from build123d import *

# Parameters (mm, degrees)
SKETCH1_R           = 7.5
BOSS_EXTRUDE1_DEPTH = 60
CUT_EXTRUDE2_DEPTH  = 60
SKETCH3_R           = 7
CUT_EXTRUDE3_DEPTH  = 104.406963015
CHAMFER1_SIZE       = 15
SPLIT2_START        = 46
SPLIT2_OUTLINE_R    = 7.5
SPLIT2_DEPTH        = 14
SPLIT2_START_2      = 52
SPLIT2_2_DEPTH      = 8
SPLIT2_3_DEPTH      = 58
SHELL1_START        = 48
SHELL1_DEPTH        = 12
SHELL1_START_2      = 54
SHELL1_2_DEPTH      = 6
CUT_EXTRUDE4_DEPTH  = 12
CUT_EXTRUDE5_DEPTH  = 6
CUT_EXTRUDE6_DEPTH  = 6


# Read off the part's stored shape, not the designer's step: Split2, Shell1
with BuildPart() as part:
    # Sketch1 → Boss-Extrude1 (new body)
    with BuildSketch(Plane(origin=(0, 0, 0), x_dir=(0, 0, -1), z_dir=(1, 0, 0))):
        with BuildLine():
            Line((-58, 0), (-58, 24))
            ThreePointArc((-58, 24), (-40.794458011, 37.276925691), (-19.581254575, 42))
            Line((-19.581254575, 42), (0, 42))
            Line((0, 42), (15, 33.339745962))
            Line((15, 33.339745962), (15, 8.660254038))
            Line((15, 8.660254038), (0, 0))
            Line((0, 0), (-58, 0))
        make_face()
        with Locations((-31, 19)):
            Circle(SKETCH1_R, mode=Mode.SUBTRACT)
    extrude(amount=BOSS_EXTRUDE1_DEPTH)

    # Sketch2 → Cut-Extrude2 (cut)
    with BuildSketch(Plane(origin=(0, 0, 0), x_dir=(1, 0, 0), z_dir=(0, 1, 0))):
        Polygon((8, -58), (30, -58), (30, -11), (14, -11), (14, -42), (8, -42), align=None)
        Polygon((30, -11), (30, -58), (52, -58), (52, -42), (46, -42), (46, -11), align=None)
    extrude(amount=CUT_EXTRUDE2_DEPTH, mode=Mode.SUBTRACT)

    # Sketch3 → Cut-Extrude3 (cut, through all)
    with BuildSketch(Plane(origin=(0, 0, -15), x_dir=(-1, 0, 0), z_dir=(0, 0, -1))):
        with Locations(Location((-30, 21, 0), (0, 0, 90))):
            Circle(SKETCH3_R)
    extrude(amount=-CUT_EXTRUDE3_DEPTH, mode=Mode.SUBTRACT)

    # Chamfer1
    chamfer1_edges = [part.edges().sort_by_distance(p)[0] for p in [
        (0, 21, -15),
        (60, 21, -15),
    ]]
    chamfer(chamfer1_edges, length=CHAMFER1_SIZE)

    # Split2 3 outline → Split2 3 (cut)
    with BuildSketch(Plane.XY):
        Polygon((60, 42), (46, 42), (46, 0), (52, 0), (60, 0), align=None)
    extrude(amount=SPLIT2_3_DEPTH, mode=Mode.SUBTRACT)


with BuildPart() as body_2:
    # Split2 outline → Split2 (new body)
    with BuildSketch(Plane.YZ.offset(SPLIT2_START)):
        with BuildLine():
            Line((0, 42), (0, 0))
            Line((0, 0), (42, 0))
            Line((42, 0), (42, 19.581254575))
            ThreePointArc((42, 19.581254575), (40.654979081, 31.100499804), (36.692279575, 42))
            Line((36.692279575, 42), (0, 42))
        make_face()
        with Locations((19, 31)):
            Circle(SPLIT2_OUTLINE_R, mode=Mode.SUBTRACT)
    extrude(amount=SPLIT2_DEPTH)

    # Split2 2 outline → Split2 2 (add)
    with BuildSketch(Plane.YZ.offset(SPLIT2_START_2)):
        with BuildLine():
            Line((0, 58), (0, 42))
            Line((0, 42), (36.692279575, 42))
            ThreePointArc((36.692279575, 42), (31.171755598, 50.654934168), (24, 58))
            Line((24, 58), (0, 58))
        make_face()
    extrude(amount=SPLIT2_2_DEPTH)

    # Shell1 outline → Shell1 (cut)
    with BuildSketch(Plane.YZ.offset(SHELL1_START)):
        with BuildLine():
            ThreePointArc((40, 19.581254575), (38.846252688, 30.042067598), (35.440474621, 40))
            Line((35.440474621, 40), (22.041381265, 40))
            ThreePointArc((22.041381265, 40), (19, 21.5), (15.958618735, 40))
            Line((15.958618735, 40), (2, 40))
            Line((2, 40), (2, 2))
            Line((2, 2), (40, 2))
            Line((40, 2), (40, 19.581254575))
        make_face()
    extrude(amount=SHELL1_DEPTH, mode=Mode.SUBTRACT)

    # Shell1 2 outline → Shell1 2 (cut)
    with BuildSketch(Plane.YZ.offset(SHELL1_START_2)):
        with BuildLine():
            Line((22.041381265, 40), (35.440474621, 40))
            ThreePointArc((35.440474621, 40), (30.201195976, 48.644437917), (23.267794641, 56))
            Line((23.267794641, 56), (2, 56))
            Line((2, 56), (2, 40))
            Line((2, 40), (15.958618735, 40))
            ThreePointArc((15.958618735, 40), (19, 40.5), (22.041381265, 40))
        make_face()
    extrude(amount=SHELL1_2_DEPTH, mode=Mode.SUBTRACT)

    # Sketch4 → Cut-Extrude4 (cut)
    with BuildSketch(Plane(origin=(48, 0, 0), x_dir=(0, 0, -1), z_dir=(1, 0, 0))):
        with BuildLine():
            Line((-40, 15.958618735), (-40, 22.041381265))
            ThreePointArc((-40, 22.041381265), (-21.5, 19), (-40, 15.958618735))
        make_face()
    extrude(amount=CUT_EXTRUDE4_DEPTH, mode=Mode.SUBTRACT)

    # Sketch5 → Cut-Extrude5 (cut)
    with BuildSketch(Plane(origin=(54, 0, 0), x_dir=(0, 0, -1), z_dir=(1, 0, 0))):
        Polygon((-40, 14.184038534), (-40, 24.39394248), (-43.350764403, 21.043178076), align=None)
    extrude(amount=CUT_EXTRUDE5_DEPTH, mode=Mode.SUBTRACT)

    # Sketch6 → Cut-Extrude6 (cut)
    with BuildSketch(Plane(origin=(60, 0, 0), x_dir=(0, 0, -1), z_dir=(1, 0, 0))):
        with BuildLine():
            ThreePointArc((-56, 23.267794641), (-57.020752822, 22.038042064), (-58, 20.77498914))
            Line((-58, 20.77498914), (-58, 2))
            Line((-58, 2), (-56, 2))
            Line((-56, 2), (-56, 23.267794641))
        make_face()
    extrude(amount=-CUT_EXTRUDE6_DEPTH, mode=Mode.SUBTRACT)


with BuildPart() as part_1:
    add(part.part)

    # Combine1: union body 2
    add(body_2.part)


solid = part_1.part
Input: part model. Units: mm. Frame: model coordinates. A direction names the side the tool comes from. Coordinates: 2 decimals unless noted, no trailing zeros. Order: outer loops, then holes, each group sorted by start corner. A loop starts at its lowest first (then second) coordinate and runs counter-clockwise, first axis right, second up. Notation, with made-up numbers: M 27.25,44 L 73.25,44 A23 cw 73.25,53 Z; hole C 42,26 d1. An arc over 180 degrees is marked long. Answer as CSV lines item,"result".
1. Section A-A (x = 30). Return the cut outline in (y, z).
Reported:
outline,"M 0,0 L 8.66,-15 L 14,-15 L 14,11 L 0,11 Z; M 28,-15 L 33.34,-15 L 42,0 L 42,11 L 28,11 Z"
2. First-contact query: P1, Ø12, axis at x = 15, y = 21.5, coming from the +Z side; P2, Ø10, axis at y = 22, z = 15.5, coming from the -X side; P3, Ø13.5, axis at y = 19, z = 31, coming from the +X side; P4, Ø2, axis at y = 16.5, z = -7, coming from the +X side. Flat tips, straight axial feed; report the tip coordinate or a pass-through.
Reported:
P1,"z = 42"
P2,"x = 0"
P3,"through"
P4,"x = 54"
3. Section D-D (z = 31). Return the cut outline in (x, y).
Reported:
outline,"M 0,0 L 14,0 L 14,11.5 L 0,11.5 Z; M 0,26.5 L 14,26.5 L 14,40.68 L 0,40.68 Z; M 46,0 L 60,0 L 60,2 L 48,2 L 48,11.5 L 46,11.5 Z; M 46,26.5 L 48,26.5 L 48,38.62 L 60,38.62 L 60,40.68 L 46,40.68 Z"
4. Section B-B (z = 4). Return the cut outline in (x, y), then the cut area to 3 significant figures.
Reported:
outline,"M 0,0 L 60,0 L 60,2 L 48,2 L 48,40 L 60,40 L 60,42 L 0,42 Z; hole C 30,21 d14"
area,"1,910 mm2"
5. Pull-direction query (Z, two-part tool) for faces 1 (the flat face through (11, 18, 42)), 2 (the cylindrical face through (6.9, 24.1, 36.5)), 3 (the cylindrical face through (46.99, 17.37, 23.68)), 4 (the flat face through (46, 21, 23)); classes: released by +Z, released by -Z, zero draft, split by the parting line, or undercut.
Reported:
face 1,"released by +Z"
face 2,"undercut"
face 3,"undercut"
face 4,"zero draft"
6. Access query for faces 5 (the flat face through (37.3, 20.7, 11)), 6 (the flat face through (29.58, 38.69, -5.73)), 7 (the flat face through (48, 21, 21)). Directions: +Z, -Z, +X, -X, +Y, -Y. A direction counts if a zero-diameter tool reaches every point of the face in a straight line with its end or side. Return the directions, or none.
Reported:
face 5,"+Z, +Y, -Y"
face 6,"-Z, +X, -X, +Y"
face 7,"+X"
7. Section C-C (y = 19). State how many separate pieces and enclosed holes the cut face has, then the cut area to 3 significant figures.
Reported:
separate pieces,"4"
enclosed holes,"0"
area,"1,310 mm2"
8. Material intervals for line 1 (X direction, y = 21, z = 0.75); line 2 (X direction, y = 11, z = 13); line 3 (X direction, y = 32, z = 3), sorted ascending. Write a range as from..to.
Reported:
line 1,"0..23, 37..60"
line 2,"0..14, 46..48"
line 3,"0..48"
